Input: dimensioned drawing with shaded views. Units: mm. Origin: part minimum x, y, z. A direction names the side the tool comes from. Coordinates: 2 decimals unless noted, no trailing zeros. Loops run counter-clockwise (first coordinate to the right, second up) from the corner with the lowest first, then second, coordinate; pieces in that order, holes last.
Item 1: Section B-B on z = 1.5. Return loops of the section in (x, y).
Item 2: Section C-C on z = 0.5. Return loops of the section in (x, y).
Item 3: Contact query for flat-ended pins moving along their axis: P1, Ø1.2, axis at y = 3, z = 1, coming from the +X side; P2, Ø0.6, axis at x = 4, z = 1, coming from the -Y side; P3, Ø1, axis at x = 0.5, z = 1, coming from the +Y side. Output: stop coordinate, or through.
Item 4: Ray query, line 1 along Z through (x, y) = (0.75, 0.35) (3 decimals); line 2 along Y through (x, z) = (4.05, 0.3); line 3 along X through (y, z) = (2.75, 1.35). Return the intervals inside material, ascending.
Item 5: Reachability of the marked faces 1, 2 and 3 from +Z, -Z, +X, -X, +Y, -Y: full face, straight path, thin tool, end or side. Return the list, or none.
Item 6: Section D-D on y = 2.25. Return loops of the section in (x, z), and give its area (4 significant figures).
Item 7: Section A-A on x = 0.75. Return loops of the section in (y, z) (3 decimals).
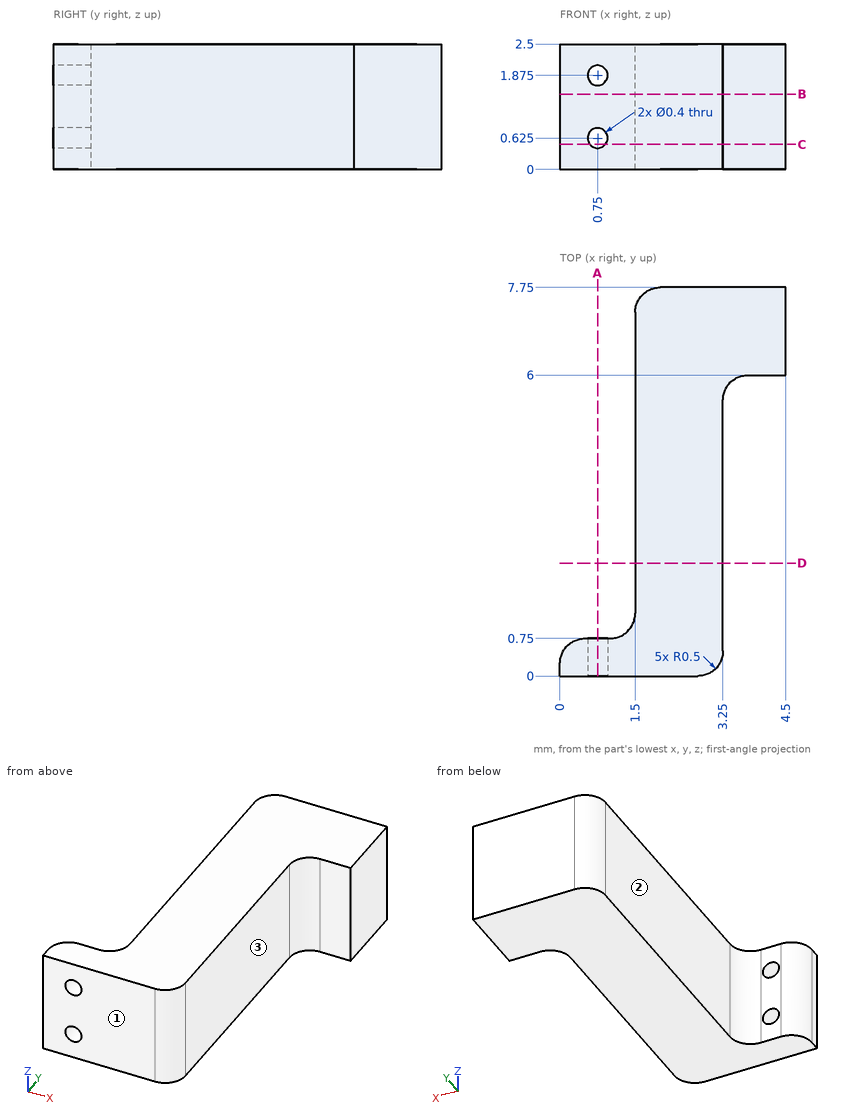
Results found:
1. outline: (0, 0) - (2.75, 0) arc R0.5 ccw to (3.25, 0.5) - (3.25, 5.5) arc R0.5 cw to (3.75, 6) - (4.5, 6) - (4.5, 7.75) - (2, 7.75) arc R0.5 ccw to (1.5, 7.25) - (1.5, 1.25) arc R0.5 cw to (1, 0.75) - (0.5, 0.75) arc R0.5 ccw to (0, 0.25) - close
2. outline: (0, 0) - (0.59, 0) - (0.59, 0.75) - (0.5, 0.75) arc R0.5 ccw to (0, 0.25) - close; (0.91, 0) - (2.75, 0) arc R0.5 ccw to (3.25, 0.5) - (3.25, 5.5) arc R0.5 cw to (3.75, 6) - (4.5, 6) - (4.5, 7.75) - (2, 7.75) arc R0.5 ccw to (1.5, 7.25) - (1.5, 1.25) arc R0.5 cw to (1, 0.75) - (0.91, 0.75) - close
3. P1: stops at x = 3.25
3. P2: stops at y = 6
3. P3: stops at y = 0.75
4. line 1: z = 0 to 0.425, 0.825 to 1.675, 2.075 to 2.5
4. line 2: y = 6 to 7.75
4. line 3: x = 1.5 to 3.25
5. face 1: +Z, -Z, +X, -X, -Y
5. face 2: +Z, -Z, -X, +Y
5. face 3: +Z, -Z, +X, -Y
6. outline: (1.5, 0) - (3.25, 0) - (3.25, 2.5) - (1.5, 2.5) - close
6. area: 4.375 mm2
7. outline: (0, 0) - (0.75, 0) - (0.75, 0.425) - (0, 0.425) - close; (0, 0.825) - (0.75, 0.825) - (0.75, 1.675) - (0, 1.675) - close; (0, 2.075) - (0.75, 2.075) - (0.75, 2.5) - (0, 2.5) - close
